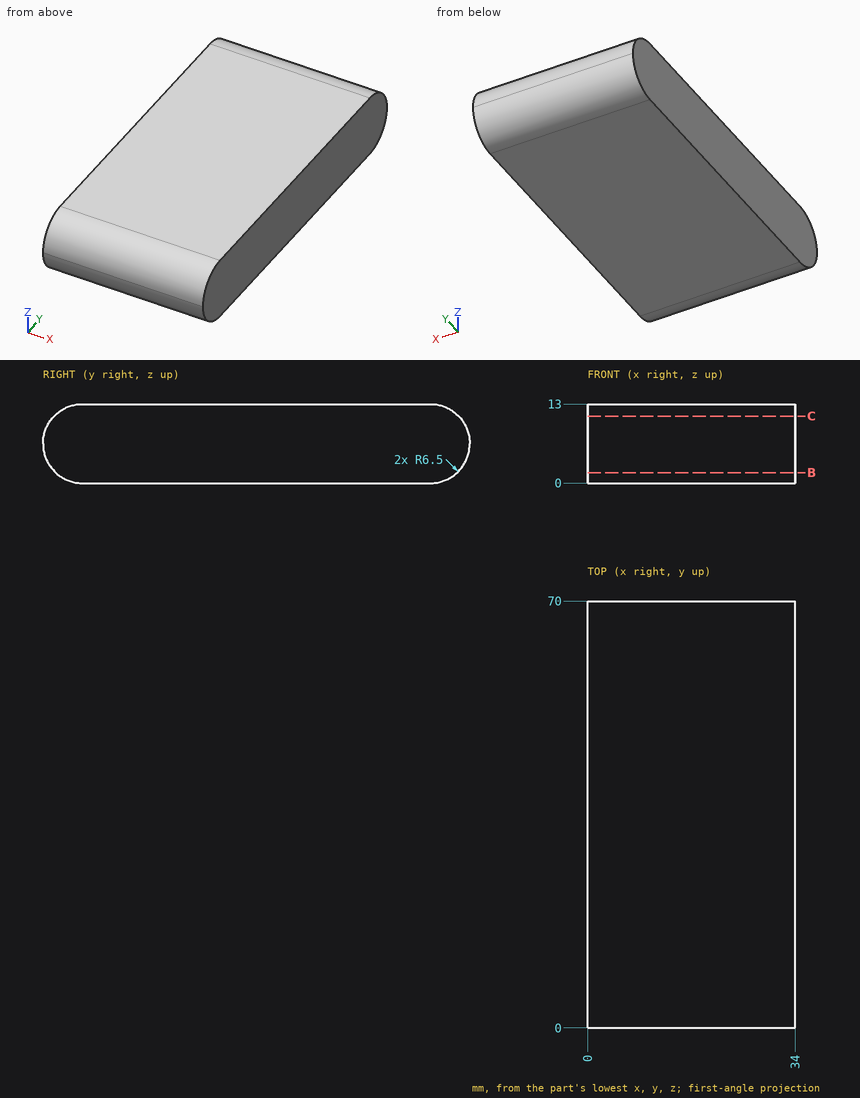
Print and shaded views of the part. All mm, measured from the part's lowest x, y and z. Give positions to 0.01 mm unless a question says otherwise; leave off trailing zeros. Loops run counter-clockwise (first coordinate to the right, second up) from the corner with the lowest first, then second, coordinate; pieces in that order, holes last. Notation, with made-up numbers: (-30, -31) - (-5, -31) arc R36 cw to (-5, 5) - close; hole circle Ø2 at (-1.75, 24). An arc over 180 degrees is marked (long way). One line per item, written item: value. Start each with the question number.
1. Slice it at B-B (z = 1.75). List the corners of the cut face in (x, y), plus the area to 3 significant figures.
2. Pin check, flat tip, straight feed: pin 1 (1.5 mm diameter, centred on x = 28, z = 11, fed in from -Y). Stop position of the tip, or through.
3. Slice it at C-C (z = 11). List the corners of the cut face in (x, y), plus the area to 3 significant figures.
4. Probe L1, parallel to Z at x = 28, y = 6; L2, parallel to Y at x = 27, z = 3.75; L3, parallel to Y at x = 21.5, z = 6. List the from-to ranges inside material, lowest first. Write a range as from..to.
Solution:
1. outline: (0, 2.06) - (34, 2.06) - (34, 67.94) - (0, 67.94) - close
1. area: 2,240 mm^2
2. pin 1: stops at y = 1.19
3. outline: (0, 1.81) - (34, 1.81) - (34, 68.19) - (0, 68.19) - close
3. area: 2,260 mm^2
4. L1: z = 0.02..12.98
4. L2: y = 0.61..69.39
4. L3: y = 0.02..69.98
